The listing builds one solid part. Answer for the finished solid, in the listing's coordinates (mm). A direction names the side the tool comes from. Give positions to 0.01 mm unless a question says otherwise; leave off trailing zeros. Write each loop counter-clockwise with the first axis right and the second up, starting at its lowest first coordinate (ties: lowest second). Pieces come first, ordered by that corner, then holes. Notation, with made-up numbers: (1, 24.5) -> (8, 24.5) arc R30 cw to (8, 49.5) -> close; hole circle Ø6 at (3.25, 76.5). An arc over 180 degrees is marked (long way). Put each result on its own line as item: value. Start each with the question number.
1) Find the intervals of material crossed by line 1 along X through (y, z) = (0.7, 0); line 2 along Y through (x, z) = (2.5, 3.25); line 3 along Y through (x, z) = (13.5, -4), in increasing order. Write a range as from..to.
2) For a pull along Z with two mould halves and no side action, classify faces 1 (the cylindrical face through (15.376, 1.268, 0.217)), 2 (the flat face through (0, -4, 6.2)), 3 (the flat face through (6, 15.5, 0)) as released by +Z, released by -Z, zero draft, split by the parting line, or undercut.
3) A cutting plane is placed at B-B (x = -14.4). Write down the section's boundary in (y, z).
4) Flat-ended cylindrical pins translate along their axes: pin 1 Ø2 at (y, z) = (-3, 6) entering from +X; pin 2 Ø8.5 at (x, y) = (5.5, -8) entering from +Z; pin 3 Ø3.5 at (x, z) = (-14.5, -2) entering from +Y. Find the tip coordinate at first contact, or state that the pin passes through.
5) For faces 4 (the flat face through (-13, 2.5, 0)), 5 (the flat face through (3, 14, 2)), 6 (the flat face through (11.4, -9, 0)), 7 (the flat face through (-13, 0, 0)), 8 (the flat face through (0, -4, -6.2)), determine the directions among +Z, -Z, +X, -X, +Y, -Y from which every point of the face is accessible in a straight line to the end or side of a thin tool.
6) A cutting plane is placed at A-A (z = 0). Write down the section's boundary in (x, y), then the cut area to 3 significant figures.
7) A cutting plane is placed at D-D (x = 5.4). Write down the section's boundary in (y, z), then the cut area to 3 significant figures.
8) A cutting plane is placed at C-C (z = -5.75). Write down the section's boundary in (x, y), then the cut area to 3 significant figures.
from build123d import *

# Parameters (mm, degrees)
SKETCH2_W           = 32.1
SKETCH2_H           = 12.4
BOSS_EXTRUDE1_DEPTH = 2.5
SKETCH3_W           = 22.8
SKETCH3_H           = 12.4
BOSS_EXTRUDE2_DEPTH = 18.5
SKETCH4_W           = 22.8
SKETCH4_H           = 12.4
BOSS_EXTRUDE3_DEPTH = 7.4
SKETCH5_R           = 2.5
BOSS_EXTRUDE4_DEPTH = 4.1
SKETCH6_R           = 1
CUT_EXTRUDE1_DEPTH  = 28.148526664
SKETCH7_R           = 10
BOSS_EXTRUDE5_DEPTH = 1.5


with BuildPart() as part:
    # Sketch2 → Boss-Extrude1 (new body)
    with BuildSketch(Plane(origin=(0, 0, 0), x_dir=(1, 0, 0), z_dir=(0, 1, 0))):
        Rectangle(SKETCH2_W, SKETCH2_H)
    extrude(amount=BOSS_EXTRUDE1_DEPTH)

    # Sketch3 → Boss-Extrude2 (add)
    with BuildSketch(Plane(origin=(0, 0, 0), x_dir=(-1, 0, 0), z_dir=(0, -1, 0))):
        Rectangle(SKETCH3_W, SKETCH3_H)
    extrude(amount=BOSS_EXTRUDE2_DEPTH)

    # Sketch4 → Boss-Extrude3 (add)
    with BuildSketch(Plane(origin=(0, 2.5, 0), x_dir=(1, 0, 0), z_dir=(0, 1, 0))):
        Rectangle(SKETCH4_W, SKETCH4_H)
    extrude(amount=BOSS_EXTRUDE3_DEPTH)

    # Sketch5 → Boss-Extrude4 (add)
    with BuildSketch(Plane(origin=(0, 9.9, 0), x_dir=(1, 0, 0), z_dir=(0, 1, 0))):
        with Locations(Location((5.4, 0, 0), (0, 0, 90))):
            Circle(SKETCH5_R)
    extrude(amount=BOSS_EXTRUDE4_DEPTH)

    # Sketch6 → Cut-Extrude1 (cut, through all)
    with BuildSketch(Plane(origin=(0, 2.5, 0), x_dir=(1, 0, 0), z_dir=(0, 1, 0))):
        with Locations(Location((-14.4, 0, 0), (0, 0, 270))):
            Circle(SKETCH6_R)
        with Locations(Location((14.4, 0, 0), (0, 0, 90))):
            Circle(SKETCH6_R)
    extrude(amount=-CUT_EXTRUDE1_DEPTH, mode=Mode.SUBTRACT)

    # Sketch7 → Boss-Extrude5 (add)
    with BuildSketch(Plane(origin=(0, 14, 0), x_dir=(1, 0, 0), z_dir=(0, 1, 0))):
        with Locations(Location((5.4, 0, 0), (0, 0, 270))):
            Circle(SKETCH7_R)
    extrude(amount=BOSS_EXTRUDE5_DEPTH)


solid = part.part
Reply:
1. line 1: x = -16.05..-15.4, -13.4..13.4, 15.4..16.05
1. line 2: y = -18.5..9.9, 14..15.5
1. line 3: y = 0..2.5, 14..15.5
2. face 1: undercut
2. face 2: released by +Z
2. face 3: zero draft
3. outline: (0, -6.2) -> (2.5, -6.2) -> (2.5, -1) -> (0, -1) -> close; (0, 1) -> (2.5, 1) -> (2.5, 6.2) -> (0, 6.2) -> close
4. pin 1: stops at x = 11.4
4. pin 2: stops at z = 6.2
4. pin 3: stops at y = 2.5
5. face 4: +Z, -Z, -X, +Y
5. face 5: none
5. face 6: +Z, -Z, +X, -Y
5. face 7: +Z, -Z, -X, -Y
5. face 8: -Z, +X, -X, -Y
6. outline: (-16.05, 0) -> (-15.4, 0) -> (-15.4, 2.5) -> (-16.05, 2.5) -> close; (-13.4, 0) -> (-11.4, 0) -> (-11.4, -18.5) -> (11.4, -18.5) -> (11.4, 0) -> (13.4, 0) -> (13.4, 2.5) -> (11.4, 2.5) -> (11.4, 9.9) -> (7.9, 9.9) -> (7.9, 14) -> (15.4, 14) -> (15.4, 15.5) -> (-4.6, 15.5) -> (-4.6, 14) -> (2.9, 14) -> (2.9, 9.9) -> (-11.4, 9.9) -> (-11.4, 2.5) -> (-13.4, 2.5) -> close; (15.4, 0) -> (16.05, 0) -> (16.05, 2.5) -> (15.4, 2.5) -> close
6. area: 711 mm2
7. outline: (-18.5, -6.2) -> (9.9, -6.2) -> (9.9, -2.5) -> (14, -2.5) -> (14, -10) -> (15.5, -10) -> (15.5, 10) -> (14, 10) -> (14, 2.5) -> (9.9, 2.5) -> (9.9, 6.2) -> (-18.5, 6.2) -> close
7. area: 403 mm2
8. outline: (-16.05, 0) -> (-11.4, 0) -> (-11.4, -18.5) -> (11.4, -18.5) -> (11.4, 0) -> (16.05, 0) -> (16.05, 2.5) -> (11.4, 2.5) -> (11.4, 9.9) -> (-11.4, 9.9) -> (-11.4, 2.5) -> (-16.05, 2.5) -> close; (-2.78, 14) -> (13.58, 14) -> (13.58, 15.5) -> (-2.78, 15.5) -> close
8. area: 695 mm2
